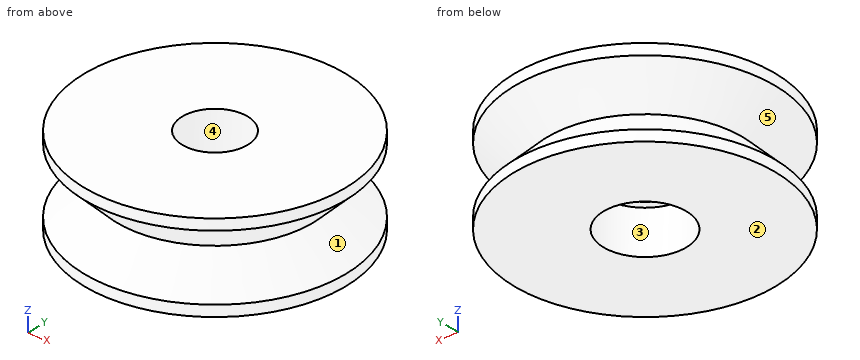
```python
from build123d import *

# Parameters (mm, degrees)
SKETCH1_R           = 6
SKETCH1_R_2         = 1.9
BOSS_EXTRUDE1_DEPTH = 2
CHAMFER1_SIZE       = 1.5
SKETCH2_R           = 6
SKETCH2_R_2         = 1.5
BOSS_EXTRUDE2_DEPTH = 2
CHAMFER2_SIZE       = 1.5


with BuildPart() as part:
    # Sketch1 → Boss-Extrude1 (new body)
    with BuildSketch(Plane.XY):
        Circle(SKETCH1_R)
        Circle(SKETCH1_R_2, mode=Mode.SUBTRACT)
    extrude(amount=BOSS_EXTRUDE1_DEPTH)

    # Chamfer1
    chamfer1_edges = [part.edges().sort_by_distance(p)[0] for p in [
        (-6, 0, 2),
    ]]
    chamfer(chamfer1_edges, length=CHAMFER1_SIZE)

    # Sketch2 → Boss-Extrude2 (add)
    with BuildSketch(Plane.XY.offset(2)):
        Circle(SKETCH2_R)
        Circle(SKETCH2_R_2, mode=Mode.SUBTRACT)
    extrude(amount=BOSS_EXTRUDE2_DEPTH)

    # Chamfer2
    chamfer2_edges = [part.edges().sort_by_distance(p)[0] for p in [
        (-6, 0, 2),
    ]]
    chamfer(chamfer2_edges, length=CHAMFER2_SIZE - 0.0001)  # a hair under: the kernel refuses the full size


solid = part.part
```
The model under review builds one solid part; all positions refer to its coordinate system, in mm. Face numbers are marked on the shaded views. A direction names the side the tool comes from. Round coordinates to 2 decimals unless told otherwise and drop trailing zeros. Write each loop counter-clockwise with the first axis right and the second up, starting at its lowest first coordinate (ties: lowest second). Pieces come first, ordered by that corner, then holes. Notation, with made-up numbers: M 18.25,46.25 L 47.25,46.25 A24 cw 47.25,82.25 Z; hole C -27,34.25 d4. An arc over 180 degrees is marked long. Use CSV: the item, a comma, the result in double quotes. Start each with the question number.
(1) We need section D-D, the plane z = 3.35. State the section outline as (x, y) points.
(2) We need section C-C, the plane z = 1.3. State the section outline as (x, y) points, then the cut area to 3 significant figures.
(3) The part is to be moulded in two halves that separate along X. For the marked faces 1, 2 and 3, say which applies: +X half, -X half, draft (parallel to the pull), parting line (faces both ways), or undercut.
(4) Tool access review of the marked faces 4 and 5: name each direction out of +Z, -Z, +X, -X, +Y, -Y from which nothing blocks a thin tool from reaching the whole face with its end or side.
(5) Clearance check with flat-ended pins moving along their axes: P1, Ø2, axis at y = 0.5, z = 2, coming from the +X side; P2, Ø2.5, axis at x = 0, y = 0, coming from the +Z side. State where each tip first meets the part, or that it passes through.
(6) For line 1 along X through (y, z) = (-1.25, 3.65); line 2 along X through (y, z) = (1, 1.5); line 3 along Z through (x, y) = (4.75, -3), list the stretches that pass through material, from the lowest coordinate up.
Findings:
1,outline,"C 0,0 d11.7; hole C 0,0 d3"
2,outline,"C 0,0 d10.4; hole C 0,0 d3.8"
2,area,"73.6 mm^2"
3,face 1,"parting line"
3,face 2,"draft"
3,face 3,"undercut"
4,face 4,"+Z, -Z"
4,face 5,"none"
5,P1,"x = 5.48"
5,P2,"through"
6,line 1,"-5.87 to -0.83, 0.83 to 5.87"
6,line 2,"-4.9 to -1.62, 1.62 to 4.9"
6,line 3,"0 to 0.88, 3.12 to 4"
